```python
from build123d import *

# Parameters (mm, degrees)
PAD_DEPTH       = 55
SKETCH001_R     = 1.6
POCKET_DEPTH    = 5.68
POCKET001_DEPTH = 2.4
SKETCH003_R     = 2.4
SKETCH003_R_2   = 1.6
PAD001_DEPTH    = 4


with BuildPart() as part:
    # Sketch → Pad (new body)
    with BuildSketch(Plane.XY):
        Polygon((2.94, -2.84), (-2.94, -2.84), (-5.44, -0.52), (-5.44, 1.16), (-2.94, 1.16), (-2.94, 2.84), (2.94, 2.84), (2.94, 1.16), (5.44, 1.16), (5.44, -0.52), align=None)
    extrude(amount=PAD_DEPTH)

    # Sketch001 (on Face6 of Pad) → Pocket (cut)
    with BuildSketch(Plane(origin=(0, 2.84, 0), x_dir=(-1, 0, 0), z_dir=(0, 1, 0))):
        with Locations((0, 48.5)):
            Circle(SKETCH001_R)
        with Locations((0, 6.5)):
            Circle(SKETCH001_R)
    extrude(amount=-POCKET_DEPTH, mode=Mode.SUBTRACT)

    # Sketch002 (on Face1 of Pocket) → Pocket001 (cut)
    with BuildSketch(Plane.XZ.offset(2.84)):
        Polygon((0, 45.186009), (2.87, 46.843005), (2.87, 50.156995), (0, 51.813991), (-2.87, 50.156995), (-2.87, 46.843005), align=None)
        Polygon((0, 3.186009), (2.87, 4.843005), (2.87, 8.156995), (0, 9.813991), (-2.87, 8.156995), (-2.87, 4.843005), align=None)
    extrude(amount=-POCKET001_DEPTH, mode=Mode.SUBTRACT)

    # Sketch003 (on Face22 of Pocket001) → Pad001 (join)
    with BuildSketch(Plane(origin=(0, 2.84, 0), x_dir=(-1, 0, 0), z_dir=(0, 1, 0))):
        with Locations((0, 6.5)):
            Circle(SKETCH003_R)
        with Locations((0, 6.5)):
            Circle(SKETCH003_R_2, mode=Mode.SUBTRACT)
        with Locations((0, 48.5)):
            Circle(SKETCH003_R)
        with Locations((0, 48.5)):
            Circle(SKETCH003_R_2, mode=Mode.SUBTRACT)
    extrude(amount=PAD001_DEPTH)


solid = part.part
```
Can you work these out from the model? Positions are in its coordinate system, mm. A direction names the side the tool comes from. Coordinates: 2 decimals unless noted, no trailing zeros. Write each loop counter-clockwise with the first axis right and the second up, starting at its lowest first coordinate (ties: lowest second). Pieces come first, ordered by that corner, then holes. Notation, with made-up numbers: M 22.25,84 L 52.25,84 A4 ccw 52.25,91 Z; hole C 1.5,39 d10. An arc over 180 degrees is marked long. Answer as CSV lines item,"result".
Item 1: Please list where these lines run through material, in increasing order: line 1 along Z through (x, y) = (0, 0.85); line 2 along Z through (x, y) = (0, 5.6); line 3 along Z through (x, y) = (0.5, -0.75).
Geometry results:
line 1,"z = 0 to 4.9, 8.1 to 46.9, 50.1 to 55"
line 2,"z = 4.1 to 4.9, 8.1 to 8.9, 46.1 to 46.9, 50.1 to 50.9"
line 3,"z = 0 to 3.47, 9.53 to 45.47, 51.53 to 55"
Item 2: We'd pull the mould along X, two halves only. Please class faces 6 (the flat face through (1, -0.44, 50)), 7 (the flat face through (-4, 1.16, 27)), 8 (the flat face through (-5.44, 0, 27)), 9 (the flat face through (4.21, -1.66, 27.12)): +X half, -X half, draft (parallel to the pull), parting line (faces both ways), or undercut.
Geometry results:
face 6,"undercut"
face 7,"draft"
face 8,"-X half"
face 9,"+X half"
Item 3: Imagine slicing it at C-C on y = 2. List the corners of the cut face in (x, z) for me, plus the area to 3 significant figures.
Geometry results:
outline,"M -2.94,0 L 2.94,0 L 2.94,55 L -2.94,55 Z; hole C 0,6.5 d3.2; hole C 0,48.5 d3.2"
area,"307 mm2"
Item 4: I'm going to push flat-ended pins straight in: P1, Ø1.3, axis at y = 2, z = 22, coming from the -X side; P2, Ø5, axis at x = 0, z = 6.5, coming from the -Y side; P3, Ø2, axis at x = 4.5, z = 16.5, coming from the +Y side. Where does each tip first touch, or does it pass through?
Geometry results:
P1,"stops at x = -2.94"
P2,"stops at y = -0.44"
P3,"stops at y = 1.16"
Item 5: Imagine slicing it at A-A on z = 22.5. List the corners of the cut face in (x, y) for me.
Geometry results:
outline,"M -5.44,-0.52 L -2.94,-2.84 L 2.94,-2.84 L 5.44,-0.52 L 5.44,1.16 L 2.94,1.16 L 2.94,2.84 L -2.94,2.84 L -2.94,1.16 L -5.44,1.16 Z"
Item 6: Imagine slicing it at D-D on x = 4.25. List the corners of the cut face in (y, z) for me, plus the area to 3 significant figures.
Geometry results:
outline,"M -1.62,0 L 1.16,0 L 1.16,55 L -1.62,55 Z"
area,"153 mm2"
Item 7: Imagine slicing it at B-B on z = 48.5. List the corners of the cut face in (x, y) for me.
Geometry results:
outline,"M -5.44,-0.52 L -2.94,-2.84 L -2.87,-2.84 L -2.87,-0.44 L -1.6,-0.44 L -1.6,6.84 L -2.4,6.84 L -2.4,2.84 L -2.94,2.84 L -2.94,1.16 L -5.44,1.16 Z; M 1.6,-0.44 L 2.87,-0.44 L 2.87,-2.84 L 2.94,-2.84 L 5.44,-0.52 L 5.44,1.16 L 2.94,1.16 L 2.94,2.84 L 2.4,2.84 L 2.4,6.84 L 1.6,6.84 Z"
Item 8: On a 3-axis mill with a long thin cutter (end or side, diameter ignored), from which of +Z, -Z, +X, -X, +Y, -Y can I reach the whole of each face in a straight line? I mean faces 1 (the flat face through (-2, 6.84, 6)), 2 (the flat face through (2.94, 2, 27)), 3 (the cylindrical face through (0.52, 4.812, 46.157)), 4 (the flat face through (-2.87, -2, 7)), 5 (the flat face through (0, 0, 55)). Say none if no direction works.
Geometry results:
face 1,"+Z, -Z, +X, -X, +Y"
face 2,"+Z, -Z, +X, +Y"
face 3,"+Y"
face 4,"-Y"
face 5,"+Z, +X, -X, +Y, -Y"
